Check sheet for the modelled part. Datum: model origin and axes. Units: mm. Round coordinates to 2 decimals unless told otherwise and drop trailing zeros. Order: outer loops, then holes, each group sorted by start corner. A loop starts at its lowest first (then second) coordinate and runs counter-clockwise, first axis right, second up. Notation, with made-up numbers: (62, 46) -> (70, 46) arc R12 ccw to (70, 57) -> close; hole circle Ø7 at (8, -31). An arc over 180 degrees is marked (long way). Answer in a Markdown table with one row per item.
Autodesk Inventor part; units mm, degrees
ref_plane "YZ Plane" through (0, 0, 0) normal (1, 0, 0) x (0, 1, 0)
ref_plane "XZ Plane" through (0, 0, 0) normal (0, 1, 0) x (-1, 0, 0)
ref_plane "XY Plane" through (0, 0, 0) normal (0, 0, 1) x (1, 0, 0)
sketch "Sketch1" plane through (0, 0, 0) normal (0, 1, 0) x (-1, 0, 0)
  circle A0 centre (0, 0) radius 13
  circle A1 centre (0, -50) radius 15.5
  circle A2 centre (0, -120) radius 23
  line L0 (0, 21.1644) -> (-48, 21.1644)
  line L1 (-50, 19.1644) -> (-50, -152.3497)
  line L2 (-48, -154.3497) -> (48, -154.3497)
  line L3 (50, -152.3497) -> (50, 19.1644)
  line L4 (48, 21.1644) -> (0, 21.1644)
  arc A3 (50, 19.1644) -> (48, 21.1644) centre (48, 19.1644) ccw
  arc A4 (-48, 21.1644) -> (-50, 19.1644) centre (-48, 19.1644) ccw
  arc A5 (-50, -152.3497) -> (-48, -154.3497) centre (-48, -152.3497) ccw
  arc A6 (48, -154.3497) -> (50, -152.3497) centre (48, -152.3497) ccw
  point P0 (50, 21.1644)
extrude "Extrusion1" add sketch "Sketch1" along normal blind 3
fillet "Fillet1" radius 1 3 edges at (13, 3, 0) (15.5, 3, -50) (23, 3, -120)
sketch "Sketch2" plane through (0, 3, 0) normal (0, 1, 0) x (1, 0, 0)
  arc A0 (-50, -19.1644) -> (-48, -21.1644) centre (-48, -19.1644) ccw
  circle A1 centre (-43, -14.1644) radius 2.5
  circle A2 centre (-43, 147.3209) radius 2.5
  circle A3 centre (42.0794, -14.1644) radius 2.5
  circle A4 centre (42.0794, 147.3209) radius 2.5
  point P0 (0, 0)
  dimension "d20" = 5
  dimension "d21" = 5
  dimension "d22" = 5
  dimension "d23" = 5
extrude "Extrusion2" cut sketch "Sketch2" against normal blind 10
sketch "Sketch3" plane through (0, 3, 0) normal (0, 1, 0) x (1, 0, 0)
  point P0 (0, 0)
equation "\"BendRadius\" = Thickness"
equation "\"BendReliefWidth\" = Thickness"
equation "\"BendReliefDepth\" = 0.5 * Thickness"
equation "\"CornerReliefSize\" = 4 * Thickness"
equation "\"MinimumRemnant\" = 2 * Thickness"
equation "\"TransitionRadius\" = BendRadius"
equation "\"JacobiRadiusSize\" = BendRadius"
equation "\"GapSize\" = Thickness"
properties part number "Circle_Color"
Item 1: Cross-section at A-A (z = -50). Record the boundary of the cut face in (x, y).
Result sheet:
| item | result |
|---|---|
| outline | (-50, 0) -> (-15.5, 0) -> (-15.5, 2) arc R1 ccw to (-16.5, 3) -> (-50, 3) -> close; (15.5, 0) -> (50, 0) -> (50, 3) -> (16.5, 3) arc R1 ccw to (15.5, 2) -> close |
Item 2: Cross-section at B-B (x = -43). Record the boundary of the cut face in (y, z).
Result sheet:
| item | result |
|---|---|
| outline | (0, -154.35) -> (3, -154.35) -> (3, -149.82) -> (0, -149.82) -> close; (0, -144.82) -> (3, -144.82) -> (3, 11.66) -> (0, 11.66) -> close; (0, 16.66) -> (3, 16.66) -> (3, 21.16) -> (0, 21.16) -> close |
Item 3: Scan lines: line 1 (Z direction, x = 0, y = 0.75); line 2 (X direction, y = 0.2, z = -146); line 3 (Z direction, x = 14, y = 2.6). Record each from-to range of solid material in increasing order. Write a range as [from, to].
Result sheet:
| item | result |
|---|---|
| line 1 | z = [-154.35, -143], [-97, -65.5], [-34.5, -13], [13, 21.16] |
| line 2 | x = [-50, -45.12], [-40.88, 39.96], [44.2, 50] |
| line 3 | z = [-154.35, -138.5], [-101.5, -57.11], [-42.89, 21.16] |
Item 4: Cross-section at D-D (y = 0.6). Record the boundary of the cut face in (x, z).
Result sheet:
| item | result |
|---|---|
| outline | (-50, -152.35) arc R2 ccw to (-48, -154.35) -> (48, -154.35) arc R2 ccw to (50, -152.35) -> (50, 19.16) arc R2 ccw to (48, 21.16) -> (-48, 21.16) arc R2 ccw to (-50, 19.16) -> close; hole circle Ø5 at (-43, -147.32); hole circle Ø5 at (-43, 14.16); hole circle Ø46 at (0, -120); hole circle Ø31 at (0, -50); hole circle Ø26 at (0, 0); hole circle Ø5 at (42.08, -147.32); hole circle Ø5 at (42.08, 14.16) |
Item 5: Mould release check, pull along Z, two halves, no side actions. Record for faces 1 (the cylindrical face through (-40.69, 1.52, 15.12)), 2 (the flat face through (12, 0, -65)): pulls with the +Z half, pulls with the -Z half, needs draft (parallel to the pull), parting line crosses it, or undercut.
Result sheet:
| item | result |
|---|---|
| face 1 | undercut |
| face 2 | needs draft |
Item 6: Cross-section at C-C (x = 0). Record the boundary of the cut face in (y, z).
Result sheet:
| item | result |
|---|---|
| outline | (0, -154.35) -> (3, -154.35) -> (3, -144) arc R1 ccw to (2, -143) -> (0, -143) -> close; (0, -97) -> (2, -97) arc R1 ccw to (3, -96) -> (3, -66.5) arc R1 ccw to (2, -65.5) -> (0, -65.5) -> close; (0, -34.5) -> (2, -34.5) arc R1 ccw to (3, -33.5) -> (3, -14) arc R1 ccw to (2, -13) -> (0, -13) -> close; (0, 13) -> (2, 13) arc R1 ccw to (3, 14) -> (3, 21.16) -> (0, 21.16) -> close |
